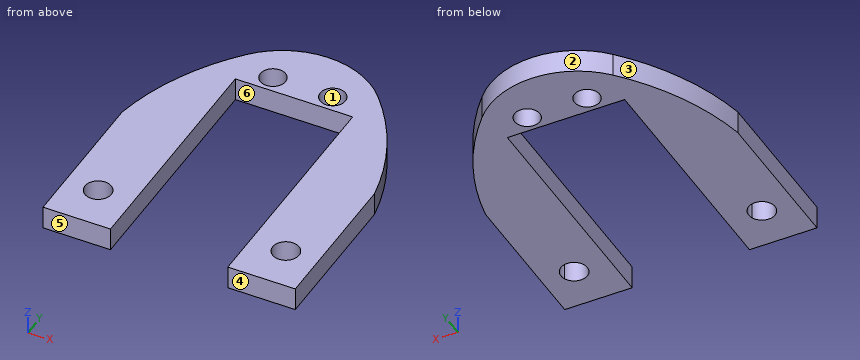
from build123d import *

# Parameters (mm, degrees)
ESQUISSE1_R             = 2.15
BOSS_EXTRU_1_DEPTH      = 4
ENL_V_MAT_EXTRU_1_DEPTH = 71.717748833
ENL_V_MAT_EXTRU_2_DEPTH = 68.644180707


with BuildPart() as part:
    # Esquisse1 → Boss.-Extru.1 (new body)
    with BuildSketch(Plane.XY):
        Polygon((0, 0), (0, 41), (-15, 56), (-28, 56), (-43, 41), (-43, 0), (-31.5, 0), (-31.5, 41), (-11.5, 41), (-11.5, 0), align=None)
        with Locations((-16.4, 43.9)):
            Circle(ESQUISSE1_R, mode=Mode.SUBTRACT)
        with Locations((-26.6, 43.9)):
            Circle(ESQUISSE1_R, mode=Mode.SUBTRACT)
    extrude(amount=BOSS_EXTRU_1_DEPTH)

    # Esquisse2 → Enlèv. mat.-Extru.1 (cut, through all)
    with BuildSketch(Plane.XY.offset(4)):
        with BuildLine():
            Line((0, 26), (0, 41))
            Line((0, 41), (-15, 56))
            Line((-15, 56), (-28, 56))
            Line((-28, 56), (-43, 41))
            Line((-43, 41), (-43, 26))
            ThreePointArc((-43, 26), (-39.293390462, 37.251091059), (-32.672201457, 47.073812699))
            ThreePointArc((-32.672201457, 47.073812699), (-21.5, 52.064721102), (-10.327798543, 47.073812699))
            ThreePointArc((-10.327798543, 47.073812699), (-3.706609538, 37.251091059), (0, 26))
        make_face()
    extrude(amount=-ENL_V_MAT_EXTRU_1_DEPTH, mode=Mode.SUBTRACT)

    # Esquisse3 → Enlèv. mat.-Extru.2 (cut, through all)
    with BuildSketch(Plane(origin=(0, 0, 0), x_dir=(-1, 0, 0), z_dir=(0, 0, -1))):
        with BuildLine():
            ThreePointArc((35.403723193, 6.682611752), (37.5, 5.25), (39.596276807, 6.682611752))
            ThreePointArc((39.596276807, 6.682611752), (37.5, 9.75), (35.403723193, 6.682611752))
        make_face()
        with BuildLine():
            ThreePointArc((7.596276807, 6.682611752), (5.5, 5.25), (3.403723193, 6.682611752))
            ThreePointArc((3.403723193, 6.682611752), (5.5, 9.75), (7.596276807, 6.682611752))
        make_face()
    extrude(amount=-ENL_V_MAT_EXTRU_2_DEPTH, mode=Mode.SUBTRACT)


solid = part.part
For this review, take the finished solid that the model builds, in its own axes (mm). Face numbers are marked on the shaded views. A direction names the side the tool comes from. Round coordinates to 2 decimals unless told otherwise and drop trailing zeros. Write each loop counter-clockwise with the first axis right and the second up, starting at its lowest first coordinate (ties: lowest second). Pieces come first, ordered by that corner, then holes. Notation, with made-up numbers: (63.25, 22.25) -> (111.25, 22.25) arc R6 cw to (111.25, 28.25) -> close; hole circle Ø11 at (33.5, 18). An arc over 180 degrees is marked (long way). Put each result on its own line as item: value.
Q1. Consider section D-D on y = 43.9. State the section outline as (x, z) points, and give its area (3 significant figures).
Determined:
outline: (-35.26, 0) -> (-28.75, 0) -> (-28.75, 4) -> (-35.26, 4) -> close; (-24.45, 0) -> (-18.55, 0) -> (-18.55, 4) -> (-24.45, 4) -> close; (-14.25, 0) -> (-7.74, 0) -> (-7.74, 4) -> (-14.25, 4) -> close
area: 75.6 mm^2
Q2. Consider section A-A on y = 7.5. State the section outline as (x, z) points.
Determined:
outline: (-43, 0) -> (-39.75, 0) -> (-39.75, 4) -> (-43, 4) -> close; (-35.25, 0) -> (-31.5, 0) -> (-31.5, 4) -> (-35.25, 4) -> close; (-11.5, 0) -> (-7.75, 0) -> (-7.75, 4) -> (-11.5, 4) -> close; (-3.25, 0) -> (0, 0) -> (0, 4) -> (-3.25, 4) -> close
Q3. Consider section B-B on z = 0.85. State the section outline as (x, y) points.
Determined:
outline: (-43, 0) -> (-31.5, 0) -> (-31.5, 41) -> (-11.5, 41) -> (-11.5, 0) -> (0, 0) -> (0, 26) arc R43.23 ccw to (-10.33, 47.07) arc R15 ccw to (-32.67, 47.07) arc R43.23 ccw to (-43, 26) -> close; hole circle Ø4.5 at (-37.5, 7.5); hole circle Ø4.3 at (-26.6, 43.9); hole circle Ø4.3 at (-16.4, 43.9); hole circle Ø4.5 at (-5.5, 7.5)
Q4. Clearance check with flat-ended pins moving along their axes: pin 1 Ø7 at (x, y) = (-5.5, 7.5) entering from -Z; pin 2 Ø1.2 at (y, z) = (30.5, 2) entering from +X. State where each tip first meets the part, or that it passes through.
Determined:
pin 1: stops at z = 0
pin 2: stops at x = -0.9
Q5. To check wall thickness, follow L1, parallel to X at y = 7.5, z = 1.85; L2, parallel to X at y = 20.5, z = 2.7; L3, parallel to Y at x = -26.6, z = 1.7. State the ranges of each line that lie inside material, in increasing order. Write a range as [from, to].
Determined:
L1: x = [-43, -39.75], [-35.25, -31.5], [-11.5, -7.75], [-3.25, 0]
L2: x = [-43, -31.5], [-11.5, 0]
L3: y = [41, 41.75], [46.05, 51.17]
Q6. Machinability: for the marked faces 5 and 6, which of the approach directions +Z, -Z, +X, -X, +Y, -Y give a long, thin tool a straight path to every point of the face, cutting with its end or side? Answer none if there is none.
Determined:
face 5: +Z, -Z, +X, -X, -Y
face 6: +Z, -Z, -Y
Q7. Consider section C-C on x = -16.4. State the section outline as (y, z) points.
Determined:
outline: (41, 0) -> (41.75, 0) -> (41.75, 4) -> (41, 4) -> close; (46.05, 0) -> (51.17, 0) -> (51.17, 4) -> (46.05, 4) -> close
Q8. The part is to be moulded in two halves that separate along X. For the marked faces 1, 2, 3 and 4, say which applies: released by +X, released by -X, zero draft, split by the parting line, or undercut.
Determined:
face 1: undercut
face 2: split by the parting line
face 3: released by -X
face 4: zero draft
